```python
from build123d import *

# Parameters (mm, degrees)
F0_R     = 5.715
F1_DEPTH = 12.7
F3_R     = 9.215
F4_DEPTH = 12.7
F5_R     = 0.5
F6_R     = 0.5


with BuildPart() as f1:
    # F0 (on Top) → F1 (new body)
    with BuildSketch(Plane.XY):
        with Locations((-0.556749, 18.462112)):
            Circle(F0_R)
    extrude(amount=F1_DEPTH)

    # F3 (on offset) → F4 (join)
    with BuildSketch(Plane.XY.offset(12.7)):
        with Locations((-0.556749, 18.462112)):
            Circle(F3_R)
    extrude(amount=F4_DEPTH)

    # F5
    f5_edges = [f1.edges().sort_by_distance(p)[0] for p in [
        (-9.771749, 18.462112, 25.4),
    ]]
    fillet(f5_edges, radius=F5_R)

    # F6
    f6_edges = [f1.edges().sort_by_distance(p)[0] for p in [
        (-6.271749, 18.462112, 0),
    ]]
    fillet(f6_edges, radius=F6_R)


solid = f1.part
```
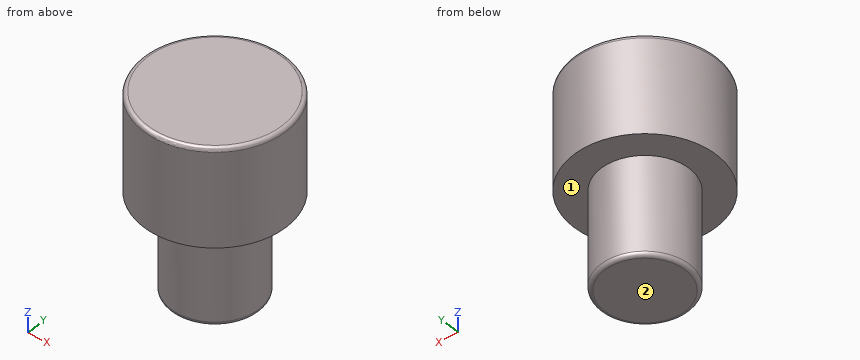
Geometry check sheet. Reference: the model listing, model coordinates, mm. Face numbers are marked on the shaded views. A direction names the side the tool comes from. Coordinates: 2 decimals unless noted, no trailing zeros. Write each loop counter-clockwise with the first axis right and the second up, starting at its lowest first coordinate (ties: lowest second). Pieces come first, ordered by that corner, then holes. Notation, with made-up numbers: (-19, 28.5) -> (33, 28.5) arc R28 ccw to (33, 53.5) -> close; hole circle Ø3 at (64.5, 74). An arc over 180 degrees is marked (long way). Use CSV: the item, a comma, the result in double quotes. Start each with the question number.
Item 1: Cross-section at A-A, the plane z = 5.25. Record the cut outline in (x, y) (3 decimals), plus the area to 3 significant figures.
Item 2: Cross-section at B-B, the plane z = 13.25. Record the cut outline in (x, y) (3 decimals), plus the area to 3 significant figures.
Item 3: Depth check by flat-ended pin: pin 1 Ø6 at (x, z) = (4.5, 6.5) entering from -Y; pin 2 Ø4 at (x, z) = (-2.5, 8) entering from +Y; pin 3 Ø5 at (y, z) = (22.5, 13) entering from -X. Enter the tip coordinate at first touch or a pass-through.
Item 4: Thickness scan on line 1 (Z direction, x = 4.5, y = 25.25); line 2 (Y direction, x = -0.75, z = 8); line 3 (Z direction, x = 4, y = 15.75). Record the ranges inside material, lowest first.
Item 5: Set-up check for the marked faces 1 and 2: record each of +Z, -Z, +X, -X, +Y, -Y from which the full face is reachable in a straight line by a thin tool's end or side.
Answers:
1,outline,"circle Ø11.43 at (-0.557, 18.462)"
1,area,"103 mm^2"
2,outline,"circle Ø18.43 at (-0.557, 18.462)"
2,area,"267 mm^2"
3,pin 1,"y = 13.13"
3,pin 2,"y = 24.18"
3,pin 3,"x = -9.64"
4,line 1,"12.7 to 25.4"
4,line 2,"12.75 to 24.17"
4,line 3,"0.01 to 25.4"
5,face 1,"-Z"
5,face 2,"-Z, +X, -X, +Y, -Y"
